```python
from build123d import *

# Parameters (mm, degrees)
SKETCH_1_W             = 30
SKETCH_1_H             = 80
EXTRUDE_1_DEPTH        = 4
SKETCH_2_R             = 1.025
CUT_EXTRUDE_1_DEPTH    = 10
PATTERN_LINEAR_1_COUNT = 5
PATTERN_LINEAR_1_PITCH = 15
SKETCH_5_W             = 30
SKETCH_5_H             = 3
EXTRUDE_3_DEPTH        = 7
FILLET_1_R             = 1
SKETCH_6_W             = 15
SKETCH_6_H             = 27
CUT_EXTRUDE_2_DEPTH    = 33
FILLET_2_R             = 2
SKETCH_7_W             = 15
SKETCH_7_H             = 30
CUT_EXTRUDE_3_DEPTH    = 33
FILLET_3_R             = 2
SKETCH_10_R            = 1.525
CUT_EXTRUDE_6_DEPTH    = 33
FILLET_5_R             = 2


with BuildPart() as part:
    # 草图1 → 凸台-拉伸1 (new body)
    with BuildSketch(Plane.XY):
        Rectangle(SKETCH_1_W, SKETCH_1_H)
    extrude(amount=EXTRUDE_1_DEPTH)

    # 草图2 → 切除-拉伸1 (cut)
    with BuildSketch(Plane.XY.offset(4)):
        with Locations((11.5, 35)):
            Circle(SKETCH_2_R)
        with Locations((-11.5, 35)):
            Circle(SKETCH_2_R)
    cut_extrude_1 = extrude(amount=-CUT_EXTRUDE_1_DEPTH, mode=Mode.SUBTRACT)

    # 阵列(线性)1: 切除-拉伸1 ×5
    with Locations(*[(0, -i * PATTERN_LINEAR_1_PITCH, 0) for i in range(1, PATTERN_LINEAR_1_COUNT)]):
        add(cut_extrude_1, mode=Mode.SUBTRACT)

    # 草图5 → 凸台-拉伸3 (add)
    with BuildSketch(Plane(origin=(0, 0, 0), x_dir=(-1, 0, 0), z_dir=(0, 0, -1))):
        with Locations((0, 1.5)):
            Rectangle(SKETCH_5_W, SKETCH_5_H)
    extrude(amount=EXTRUDE_3_DEPTH)

    # 圆角1
    fillet_1_edges = [part.edges().sort_by_distance(p)[0] for p in [
        (15, -40, 2),
        (-15, -40, 2),
        (-15, 40, 2),
        (15, 40, 2),
    ]]
    fillet(fillet_1_edges, radius=FILLET_1_R)

    # 草图6 → 切除-拉伸2 (cut, symmetric)
    with BuildSketch(Plane(origin=(0, 0, 0), x_dir=(-1, 0, 0), z_dir=(0, 0, -1))):
        with Locations((0, 21.5)):
            Rectangle(SKETCH_6_W, SKETCH_6_H)
    extrude(amount=CUT_EXTRUDE_2_DEPTH, both=True, mode=Mode.SUBTRACT)

    # 圆角2
    fillet_2_edges = [part.edges().sort_by_distance(p)[0] for p in [
        (-7.5, 35, 2),
        (-7.5, 8, 2),
        (7.5, 8, 2),
        (7.5, 35, 2),
    ]]
    fillet(fillet_2_edges, radius=FILLET_2_R)

    # 草图7 → 切除-拉伸3 (cut, symmetric)
    with BuildSketch(Plane(origin=(0, 0, 0), x_dir=(-1, 0, 0), z_dir=(0, 0, -1))):
        with Locations((0, -20)):
            Rectangle(SKETCH_7_W, SKETCH_7_H)
    extrude(amount=CUT_EXTRUDE_3_DEPTH, both=True, mode=Mode.SUBTRACT)

    # 圆角3
    fillet_3_edges = [part.edges().sort_by_distance(p)[0] for p in [
        (-7.5, -5, 2),
        (-7.5, -35, 2),
        (7.5, -35, 2),
        (7.5, -5, 2),
    ]]
    fillet(fillet_3_edges, radius=FILLET_3_R)

    # 草图10 → 切除-拉伸6 (cut, symmetric)
    with BuildSketch(Plane(origin=(0, 3, 0), x_dir=(1, 0, 0), z_dir=(0, 1, 0))):
        with Locations(Location((11, 4, 0), (0, 0, 270))):
            Circle(SKETCH_10_R)
        with Locations(Location((-11, 4, 0), (0, 0, 270))):
            Circle(SKETCH_10_R)
    extrude(amount=CUT_EXTRUDE_6_DEPTH, both=True, mode=Mode.SUBTRACT)

    # 圆角5
    fillet_5_edges = [part.edges().sort_by_distance(p)[0] for p in [
        (15, 1.5, -7),
        (-15, 1.5, -7),
    ]]
    fillet(fillet_5_edges, radius=FILLET_5_R)


solid = part.part
```
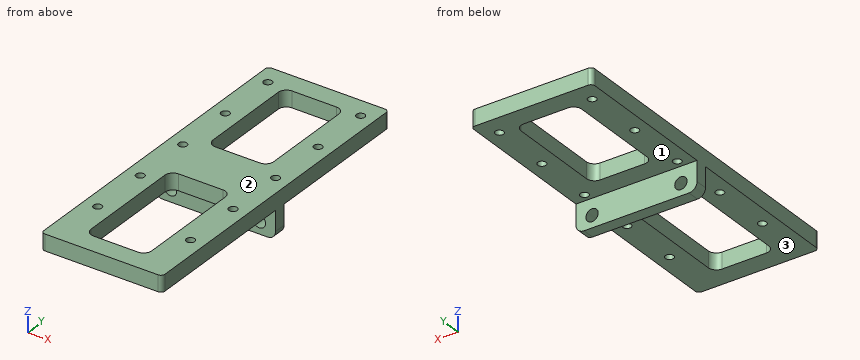
Can you work these out from the model? Positions are in its coordinate system, mm. Face numbers are marked on the shaded views. A direction names the side the tool comes from. Coordinates: 2 decimals unless noted, no trailing zeros. Order: outer loops, then holes, each group sorted by start corner. A loop starts at its lowest first (then second) coordinate and runs counter-clockwise, first axis right, second up.
1. I need wall thicknesses on line 1 (Y direction, x = 11.5, z = 1.5) (3 decimals); line 2 (X direction, y = 2, z = -4) (3 decimals); line 3 (Y direction, x = -3.25, z = 3). Which ranges of each line are inside material? Lowest first, please.
2. I'm going to push flat-ended pins straight in: pin 1 (3.5 mm diameter, centred on x = -11.5, y = 5, fed in from +Z); pin 2 (3 mm diameter, centred on x = -4.5, y = 9, fed in from -Z); pin 3 (5 mm diameter, centred on x = -3, z = -3, fed in from -Y); pin 4 (5 mm diameter, centred on x = 11, z = -4, fed in from +Y). Where does each tip first touch, or does it pass through?
3. If we section it at A-A (y = -10): Please give me the cut outline in (x, z) (3 decimals), then the cut area to 3 significant figures.
4. For the marked faces 1, 2 and 3, which set-ups out of +Z, -Z, +X, -X, +Y, -Y let a thin tool reach every point of the face, with its end or its side?
5. If we section it at C-C (z = 1.5): Give the number of separate pieces and of enclosed holes in the cut face, then the cut area to 3 significant figures.
6. If we section it at B-B (y = -29.5): Please give me the cut outline in (x, z).
7. If we section it at D-D (x = 2.25): Please give me the cut outline in (y, z), then the cut area to 3 significant figures.
Entries:
1. line 1: y = -40 to -26.025, -23.975 to -11.025, -8.975 to 3.975, 6.025 to 18.975, 21.025 to 33.975, 36.025 to 40
1. line 2: x = -15 to -12.525, -9.475 to 9.475, 12.525 to 15
1. line 3: y = -40 to -35, -5 to 8, 35 to 40
2. pin 1: stops at z = 4
2. pin 2: stops at z = 0
2. pin 3: stops at y = 0
2. pin 4: stops at y = 3
3. outline: (-15, 0) - (-12.525, 0) - (-12.525, 4) - (-15, 4) - close; (-10.475, 0) - (-7.5, 0) - (-7.5, 4) - (-10.475, 4) - close; (7.5, 0) - (10.475, 0) - (10.475, 4) - (7.5, 4) - close; (12.525, 0) - (15, 0) - (15, 4) - (12.525, 4) - close
3. area: 43.6 mm2
4. face 1: -Z, +X, -X, +Y
4. face 2: +Z, +X, -X, +Y, -Y
4. face 3: -Z, +X, -X, -Y
5. separate pieces: 1
5. enclosed holes: 12
5. area: 1,520 mm2
6. outline: (-15, 0) - (-7.5, 0) - (-7.5, 4) - (-15, 4) - close; (7.5, 0) - (15, 0) - (15, 4) - (7.5, 4) - close
7. outline: (-40, 0) - (-35, 0) - (-35, 4) - (-40, 4) - close; (-5, 0) - (0, 0) - (0, -7) - (3, -7) - (3, 0) - (8, 0) - (8, 4) - (-5, 4) - close; (35, 0) - (40, 0) - (40, 4) - (35, 4) - close
7. area: 113 mm2
